Here's how the part is built. I have some questions about the finished solid (model axes, mm). Face numbers are marked on the shaded views. A direction names the side the tool comes from. Give positions to 0.01 mm unless a question says otherwise; leave off trailing zeros. Loops run counter-clockwise (first coordinate to the right, second up) from the corner with the lowest first, then second, coordinate; pieces in that order, holes last.
Q1. Suppose I cut it at A-A (z = 18). List the corners of the cut face in (x, y) for me, and give its area (3 significant figures).
Q2. Thinking about a two-plate mould opening in Y: for the marked faces 3, 4, 5 and 6, which applies, pulls with the +Y half, pulls with the -Y half, needs draft (parallel to the pull), parting line crosses it, or undercut?
Q3. Suppose I cut it at D-D (z = -94). List the corners of the cut face in (x, y) for me.
Q4. Suppose I cut it at B-B (y = 9). List the corners of the cut face in (x, z) for me.
Q5. For the marked faces 1 and 2, which set-ups out of +Z, -Z, +X, -X, +Y, -Y let a thin tool reach every point of the face, with its end or its side?
Q6. Suppose I cut it at C-C (x = 6.75). List the corners of the cut face in (y, z) for me, and give its area (3 significant figures).
Q7. I need wall thicknesses on probe 1 along Z at (x, y) = (11.9, -6); probe 2 along Y at (x, z) = (4.5, 37.5); probe 3 along X at (y, z) = (17.5, 47). Which ranges of each line are inside material? Lowest first, please.
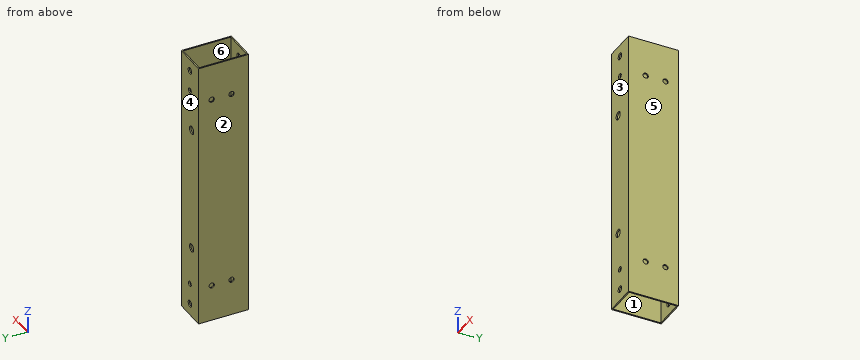
```python
from build123d import *

# Parameters (mm, degrees)
SKETCH_1_W          = 25
SKETCH_1_H          = 38
SKETCH_1_W_2        = 23
SKETCH_1_H_2        = 36
EXTRUDE_1_DEPTH     = 103
SKETCH_2_R          = 2.5
SKETCH_2_R_2        = 2
CUT_EXTRUDE_1_DEPTH = 40
SKETCH_4_R          = 3
CUT_EXTRUDE_2_DEPTH = 38
SKETCH_5_R          = 2
CUT_EXTRUDE_3_DEPTH = 108.680081724


with BuildPart() as part:
    # 草图1 → 凸台-拉伸1 (new, symmetric)
    with BuildSketch(Plane.XY):
        Rectangle(SKETCH_1_W, SKETCH_1_H)
        Rectangle(SKETCH_1_W_2, SKETCH_1_H_2, mode=Mode.SUBTRACT)
    extrude(amount=EXTRUDE_1_DEPTH, both=True)

    # 草图2 → 切除-拉伸1 (cut)
    with BuildSketch(Plane(origin=(0, 19, 0), x_dir=(1, 0, 0), z_dir=(0, 1, 0))):
        with Locations(Location((0, 94, 0), (0, 0, 270))):
            Circle(SKETCH_2_R)
        with Locations(Location((0, 78, 0), (0, 0, 270))):
            Circle(SKETCH_2_R_2)
    cut_extrude_1 = extrude(amount=-CUT_EXTRUDE_1_DEPTH, mode=Mode.SUBTRACT)

    # 镜向1: 切除-拉伸1 across plane
    add(cut_extrude_1.mirror(Plane.XY), mode=Mode.SUBTRACT)

    # 草图4 → 切除-拉伸2 (cut)
    with BuildSketch(Plane(origin=(0, 19, 0), x_dir=(1, 0, 0), z_dir=(0, 1, 0))):
        with Locations(Location((-2.5, 47.5, 0), (0, 0, 270))):
            Circle(SKETCH_4_R)
        with Locations(Location((-2.5, -47.5, 0), (0, 0, 270))):
            Circle(SKETCH_4_R)
    extrude(amount=-CUT_EXTRUDE_2_DEPTH, mode=Mode.SUBTRACT)

    # 草图5 → 切除-拉伸3 (cut, through all)
    with BuildSketch(Plane(origin=(12.5, 0, 0), x_dir=(0, 0, -1), z_dir=(1, 0, 0))):
        with Locations(Location((-75, 9, 0), (0, 0, 90))):
            Circle(SKETCH_5_R)
        with Locations(Location((-75, -6, 0), (0, 0, 90))):
            Circle(SKETCH_5_R)
        with Locations(Location((75, -6, 0), (0, 0, 90))):
            Circle(SKETCH_5_R)
        with Locations(Location((75, 9, 0), (0, 0, 90))):
            Circle(SKETCH_5_R)
    extrude(amount=-CUT_EXTRUDE_3_DEPTH, mode=Mode.SUBTRACT)


solid = part.part
```
Solutions:
1. outline: (-12.5, -19) - (12.5, -19) - (12.5, 19) - (-12.5, 19) - close; hole (-11.5, -18) - (11.5, -18) - (11.5, 18) - (-11.5, 18) - close
1. area: 122 mm2
2. face 3: pulls with the -Y half
2. face 4: pulls with the +Y half
2. face 5: needs draft
2. face 6: undercut
3. outline: (-12.5, -19) - (-2.5, -19) - (-2.5, -18) - (-11.5, -18) - (-11.5, 18) - (-2.5, 18) - (-2.5, 19) - (-12.5, 19) - close; (2.5, -19) - (12.5, -19) - (12.5, 19) - (2.5, 19) - (2.5, 18) - (11.5, 18) - (11.5, -18) - (2.5, -18) - close
4. outline: (-12.5, -103) - (-11.5, -103) - (-11.5, -77) - (-12.5, -77) - close; (-12.5, -73) - (-11.5, -73) - (-11.5, 73) - (-12.5, 73) - close; (-12.5, 77) - (-11.5, 77) - (-11.5, 103) - (-12.5, 103) - close; (11.5, -103) - (12.5, -103) - (12.5, -77) - (11.5, -77) - close; (11.5, -73) - (12.5, -73) - (12.5, 73) - (11.5, 73) - close; (11.5, 77) - (12.5, 77) - (12.5, 103) - (11.5, 103) - close
5. face 1: +Z, -Z
5. face 2: +Z, -Z, -X, +Y, -Y
6. outline: (-19, -103) - (-18, -103) - (-18, 103) - (-19, 103) - close; (18, -103) - (19, -103) - (19, 103) - (18, 103) - close
6. area: 412 mm2
7. probe 1: z = -103 to -77, -73 to 73, 77 to 103
7. probe 2: y = -19 to -18, 18 to 19
7. probe 3: x = -12.5 to -11.5, 11.5 to 12.5
